Part print with two shaded views. Sizes in mm from the minimum x, y, z corner. A direction names the side the tool comes from. Coordinates: 2 decimals unless noted, no trailing zeros. Order: outer loops, then holes, each group sorted by start corner. A loop starts at its lowest first (then second) coordinate and runs counter-clockwise, first axis right, second up. Notation, with made-up numbers: M 34.5,-39.75 L 64.5,-39.75 A20 cw 64.5,-34.75 Z; hole C 88.25,-33.75 d2. An arc over 180 degrees is marked long. Answer in a Markdown table with one row per item. Add a question column.
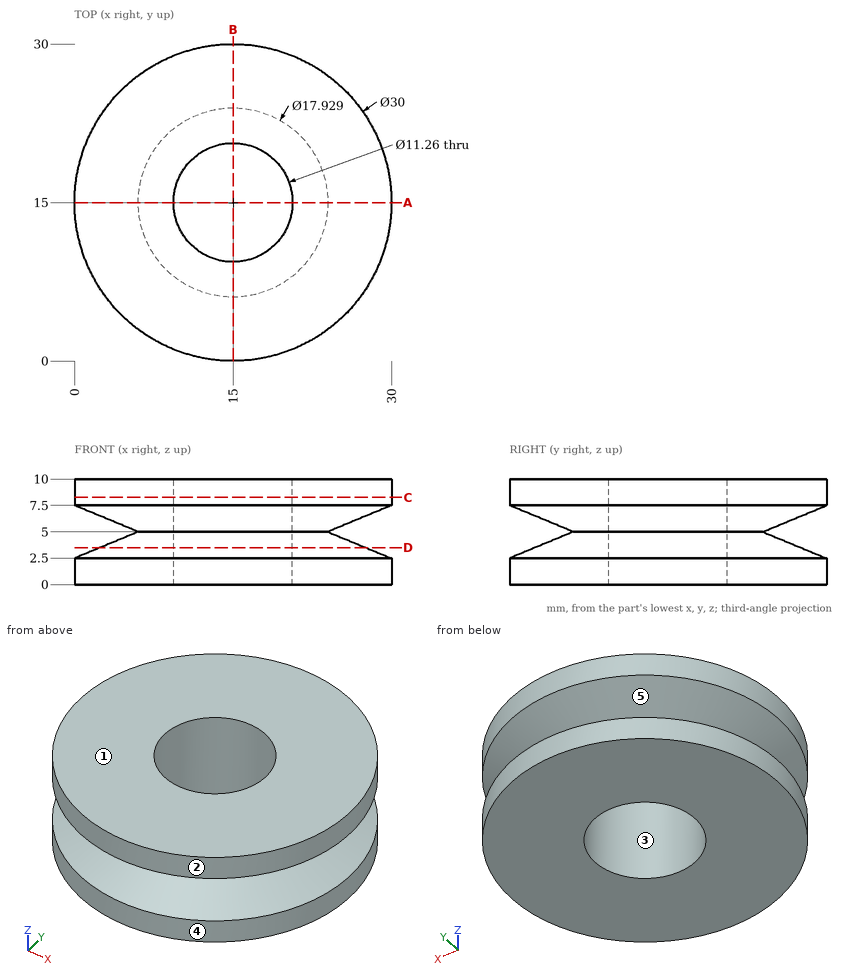
(1) Pull direction X, two halves, no side cores. Call the marked faces 1, 2 and 3: pulls with the +X half, pulls with the -X half, needs draft (parallel to the pull), parting line crosses it, or undercut.
(2) Drop flat-ended pins along their axis: P1, Ø1.5, axis at x = 15.5, z = 3.5, coming from the -Y side; P2, Ø6, axis at x = 21, z = 7, coming from the +Y side; P3, Ø5, axis at x = 4, z = 7, coming from the -Y side. Give the stop position or say it passes through.
(3) Slice it at C-C (z = 8.25). List the corners of the cut face in (x, y).
(4) Wall check: line 1 (Y direction, x = 11.5, z = 2.75) (1 decimal); line 2 (Z direction, x = 25.75, y = 21.5); line 3 (Z direction, x = 5.75, y = 24.5). Give the ranges that are in metal, low to high.
(5) Slice it at A-A (y = 15). List the corners of the cut face in (x, z), and give its area (3 significant figures).
(6) Slice it at D-D (z = 3.5). List the corners of the cut face in (x, y).
(7) 3-axis set-ups, long thin cutter, end or side, ignore diameter. For the marked faces 4 and 5: which of +Z, -Z, +X, -X, +Y, -Y reach the whole face in a straight line?
Computed:
| question | item | result |
|---|---|---|
| 1 | face 1 | needs draft |
| 1 | face 2 | parting line crosses it |
| 1 | face 3 | undercut |
| 2 | P1 | stops at y = 0.61 |
| 2 | P2 | stops at y = 29.69 |
| 2 | P3 | stops at y = 2.68 |
| 3 | outline | C 15,15 d30; hole C 15,15 d11.26 |
| 4 | line 1 | y = 1 to 10.6, 19.4 to 29 |
| 4 | line 2 | z = 0 to 3.51, 6.49 to 10 |
| 4 | line 3 | z = 0 to 3.22, 6.78 to 10 |
| 5 | outline | M 0,0 L 9.37,0 L 9.37,10 L 0,10 L 0,7.5 L 6.04,5 L 0,2.5 Z; M 20.63,0 L 30,0 L 30,2.5 L 23.96,5 L 30,7.5 L 30,10 L 20.63,10 Z |
| 5 | area | 157 mm^2 |
| 6 | outline | C 15,15 d25.17; hole C 15,15 d11.26 |
| 7 | face 4 | +Z, -Z |
| 7 | face 5 | none |
